Source: CAD feature listing. Evaluate the final solid. Frame: model axes, mm. Give positions to 0.01 mm unless a question says otherwise; leave off trailing zeros. Loops run counter-clockwise (first coordinate to the right, second up) from the corner with the lowest first, then second, coordinate; pieces in that order, holes last. Notation, with made-up numbers: (-34.5, -34) -> (-14.5, -34) arc R13 ccw to (-14.5, -9) -> close; hole circle Ø5 at (26, 18). An arc over 180 degrees is marked (long way). Put each result on its own line as item: value.
```python
from build123d import *

# Parameters (mm, degrees)
SKETCH1_W           = 97.282
SKETCH1_H           = 53.34
BOSS_EXTRUDE1_DEPTH = 2.54
SKETCH2_R           = 1.651
CUT_EXTRUDE1_DEPTH  = 56.530958762


with BuildPart() as part:
    # Sketch1 → Boss-Extrude1 (new body)
    with BuildSketch(Plane(origin=(0, 0, 0), x_dir=(1, 0, 0), z_dir=(0, 1, 0))):
        Rectangle(SKETCH1_W, SKETCH1_H)
    extrude(amount=BOSS_EXTRUDE1_DEPTH)

    # Sketch2 → Cut-Extrude1 (cut, through all)
    with BuildSketch(Plane(origin=(0, 2.54, 0), x_dir=(1, 0, 0), z_dir=(0, 1, 0))):
        with Locations(Location((-34.671, 20.32, 0), (0, 0, 270))):
            Circle(SKETCH2_R)
        with BuildLine():
            ThreePointArc((-4.137168556, 10.430937018), (-5.273705168, 8.313889423), (-7.666216208, 8.091410411))
            Line((-7.666216208, 8.091410411), (-27.062123692, 16.291136246))
            ThreePointArc((-27.062123692, 16.291136246), (-28.190123635, 17.227199464), (-28.61307604, 18.630662853))
            Line((-28.61307604, 18.630662853), (-28.61307604, 20.32))
            Line((-28.61307604, 20.32), (-6.677168556, 20.32))
            ThreePointArc((-6.677168556, 20.32), (-4.881117332, 19.576051224), (-4.137168556, 17.78))
            Line((-4.137168556, 17.78), (-4.137168556, 10.430937018))
        make_face()
        with BuildLine():
            Line((-34.671, 10.20811999), (-34.671, -10.20811999))
            ThreePointArc((-34.671, -10.20811999), (-33.552342054, -12.313205919), (-31.181719082, -12.564062634))
            Line((-31.181719082, -12.564062634), (-5.847021287, -2.355942643))
            ThreePointArc((-5.847021287, -2.355942643), (-4.256302206, 0), (-5.847021287, 2.355942643))
            Line((-5.847021287, 2.355942643), (-31.181719082, 12.564062634))
            ThreePointArc((-31.181719082, 12.564062634), (-33.552342054, 12.313205919), (-34.671, 10.20811999))
        make_face()
        with BuildLine():
            ThreePointArc((-28.61307604, -18.630662853), (-28.190123635, -17.227199464), (-27.062123692, -16.291136246))
            Line((-27.062123692, -16.291136246), (-7.666216208, -8.091410411))
            ThreePointArc((-7.666216208, -8.091410411), (-5.273705168, -8.313889423), (-4.137168556, -10.430937018))
            Line((-4.137168556, -10.430937018), (-4.137168556, -17.78))
            ThreePointArc((-4.137168556, -17.78), (-4.881117332, -19.576051224), (-6.677168556, -20.32))
            Line((-6.677168556, -20.32), (-28.61307604, -20.32))
            Line((-28.61307604, -20.32), (-28.61307604, -18.630662853))
        make_face()
        with BuildLine():
            ThreePointArc((4.137168556, -10.430937018), (5.273705168, -8.313889423), (7.666216208, -8.091410411))
            Line((7.666216208, -8.091410411), (27.062123692, -16.291136246))
            ThreePointArc((27.062123692, -16.291136246), (28.190123635, -17.227199464), (28.61307604, -18.630662853))
            Line((28.61307604, -18.630662853), (28.61307604, -20.32))
            Line((28.61307604, -20.32), (6.677168556, -20.32))
            ThreePointArc((6.677168556, -20.32), (4.881117332, -19.576051224), (4.137168556, -17.78))
            Line((4.137168556, -17.78), (4.137168556, -10.430937018))
        make_face()
        with BuildLine():
            Line((34.671, 10.20811999), (34.671, -10.20811999))
            ThreePointArc((34.671, -10.20811999), (33.552342054, -12.313205919), (31.181719082, -12.564062634))
            Line((31.181719082, -12.564062634), (5.847021287, -2.355942643))
            ThreePointArc((5.847021287, -2.355942643), (4.256302206, 0), (5.847021287, 2.355942643))
            Line((5.847021287, 2.355942643), (31.181719082, 12.564062634))
            ThreePointArc((31.181719082, 12.564062634), (33.552342054, 12.313205919), (34.671, 10.20811999))
        make_face()
        with BuildLine():
            ThreePointArc((4.137168556, 17.78), (4.881117332, 19.576051224), (6.677168556, 20.32))
            Line((6.677168556, 20.32), (28.61307604, 20.32))
            Line((28.61307604, 20.32), (28.61307604, 18.630662853))
            ThreePointArc((28.61307604, 18.630662853), (28.190123635, 17.227199464), (27.062123692, 16.291136246))
            Line((27.062123692, 16.291136246), (7.666216208, 8.091410411))
            ThreePointArc((7.666216208, 8.091410411), (5.273705168, 8.313889423), (4.137168556, 10.430937018))
            Line((4.137168556, 10.430937018), (4.137168556, 17.78))
        make_face()
        with Locations(Location((34.671, 20.32, 0), (0, 0, 270))):
            Circle(SKETCH2_R)
        with Locations(Location((34.671, -20.32, 0), (0, 0, 270))):
            Circle(SKETCH2_R)
        with Locations(Location((-34.671, -20.32, 0), (0, 0, 90))):
            Circle(SKETCH2_R)
    extrude(amount=-CUT_EXTRUDE1_DEPTH, mode=Mode.SUBTRACT)


solid = part.part
```
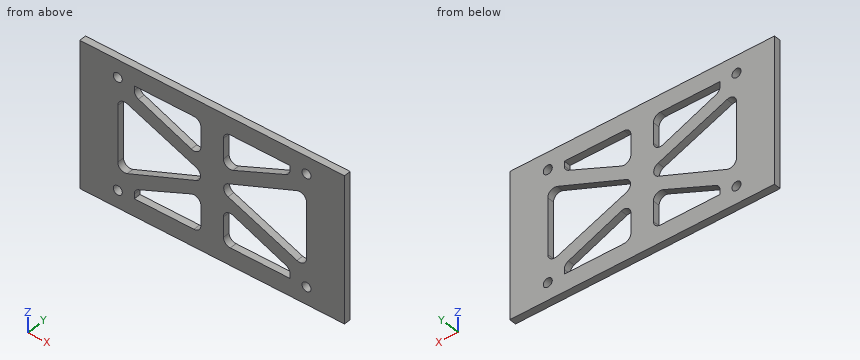
(1) Section B-B on z = -6.5. Return loops of the section in (x, y).
Calculated:
outline: (-48.64, 0) -> (-34.67, 0) -> (-34.67, 2.54) -> (-48.64, 2.54) -> close; (-16.13, 0) -> (16.13, 0) -> (16.13, 2.54) -> (-16.13, 2.54) -> close; (34.67, 0) -> (48.64, 0) -> (48.64, 2.54) -> (34.67, 2.54) -> close
(2) Line query: probe 1 along X at (y, z) = (1.55, 4.5); probe 2 along Z at (x, y) = (6.5, 0.55); probe 3 along Z at (x, y) = (-23.5, 0.95). Output: solid intervals per line, ascending. Write a range as from..to.
Calculated:
probe 1: x = -48.64..-34.67, -11.17..11.17, 34.67..48.64
probe 2: z = -26.67..-20.31, -7.9..-2.62, 2.62..7.9, 20.31..26.67
probe 3: z = -26.67..-20.32, -14.79..-9.47, 9.47..14.79, 20.32..26.67
(3) Section A-A on x = 16.5. Return loops of the section in (y, z), then the cut area to 3 significant figures.
Calculated:
outline: (0, -26.67) -> (2.54, -26.67) -> (2.54, -20.32) -> (0, -20.32) -> close; (0, -11.83) -> (2.54, -11.83) -> (2.54, -6.65) -> (0, -6.65) -> close; (0, 6.65) -> (2.54, 6.65) -> (2.54, 11.83) -> (0, 11.83) -> close; (0, 20.32) -> (2.54, 20.32) -> (2.54, 26.67) -> (0, 26.67) -> close
area: 58.6 mm²
(4) Section C-C on y = 1.9. Give the number of separate pieces and of enclosed holes in the cut face, then the cut area to 3 significant figures.
Calculated:
separate pieces: 1
enclosed holes: 10
area: 3,400 mm²
